Could you check a few things on this model? Use its own coordinates, in mm. Face numbers are marked on the shaded views. A direction names the side the tool comes from. Give positions to 0.01 mm unless a question says otherwise; leave off trailing zeros. Loops run counter-clockwise (first coordinate to the right, second up) from the corner with the lowest first, then second, coordinate; pieces in that order, holes last. Notation, with made-up numbers: (86.25, 18.25) - (139.25, 18.25) arc R11 cw to (139.25, 36.25) - close; hole circle Ø1 at (-38, 79.5). An arc over 180 degrees is marked (long way). Write each question's results on one line, items separated by ' | '. Start each with the question number.
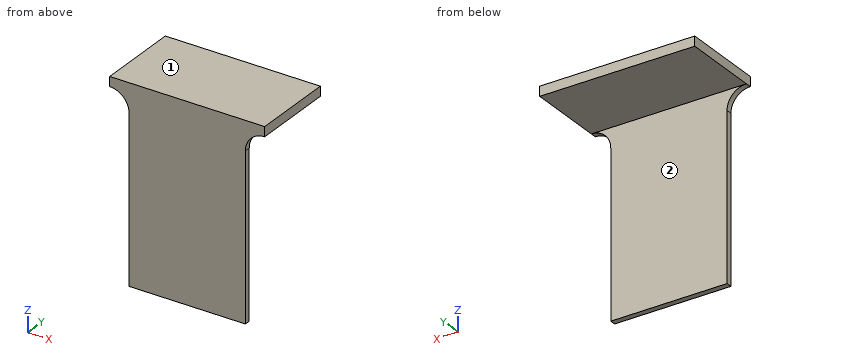
```python
from build123d import *

# Parameters (mm, degrees)
SKETCH_1_W           = 60
SKETCH_1_H           = 100
EXTRUDE_1_DEPTH      = 3
EXTRUDE_2_DEPTH      = 40
EXTRUDE_2_DEPTH_BACK = 3
SKETCH_2_W           = 80
SKETCH_2_H           = 5
FILLET_1_R           = 10


with BuildPart() as part:
    # Эскиз1 → Бобышка-Вытянуть1 (new body)
    with BuildSketch(Plane(origin=(0, 0, 0), x_dir=(1, 0, 0), z_dir=(0, 1, 0))):
        Rectangle(SKETCH_1_W, SKETCH_1_H)
    extrude(amount=EXTRUDE_1_DEPTH)

    # Эскиз2 → Бобышка-Вытянуть2 (add, two sides: drawn at the far end of the back side and taken through both)
    with BuildSketch(Plane(origin=(0, 3, 0), x_dir=(1, 0, 0), z_dir=(0, 1, 0)).offset(-EXTRUDE_2_DEPTH_BACK)):
        with Locations((0, -47.5)):
            Rectangle(SKETCH_2_W, SKETCH_2_H)
    extrude(amount=EXTRUDE_2_DEPTH + EXTRUDE_2_DEPTH_BACK)

    # Скругление1
    fillet_1_edges = [part.edges().sort_by_distance(p)[0] for p in [
        (30, 1.5, 45),
        (-30, 1.5, 45),
    ]]
    fillet(fillet_1_edges, radius=FILLET_1_R - 0.0001)  # a hair under: the kernel refuses the full size


solid = part.part
```
Q1. Which directions (+Z, -Z, +X, -X, +Y, -Y) give clear straight access to the entire face, cutting with the end or side of a thin tool? Please do the marked faces 1 and 2.
Q2. I want a section at C-C, the plane z = 26.5. List the corners of the cut face in (x, y) for me, then the cut area to 3 significant figures.
Q3. I need wall thicknesses on L1, parallel to Z at x = 29.5, y = 36.5; L2, parallel to Y at x = -7.5, z = 1. Which ranges of each line are inside material? Lowest first, please. Write a range as from..to.
Q4. I want a section at B-B, the plane y = 39.5. List the corners of the cut face in (x, z) for me.
Q5. I want a section at A-A, the plane x = 0. List the corners of the cut face in (y, z) for me.
Q6. I'm going to push flat-ended pins straight in: pin 1 Ø2 at (x, z) = (13, -28.5) entering from -Y; pin 2 Ø6 at (x, y) = (-17.5, 16) entering from -Z; pin 3 Ø3.5 at (y, z) = (2, 12) entering from +X; pin 4 Ø8 at (x, z) = (-7.5, -2) entering from +Y. Where does each tip first touch, or does it pass through?
Conclusion:
1) face 1: +Z, +X, -X, +Y, -Y | face 2: -Z, +X, -X, +Y
2) outline: (-30, 0) - (30, 0) - (30, 3) - (-30, 3) - close | area: 180 mm^2
3) L1: 45..50 | L2: 0..3
4) outline: (-40, 45) - (40, 45) - (40, 50) - (-40, 50) - close
5) outline: (0, -50) - (3, -50) - (3, 45) - (43, 45) - (43, 50) - (0, 50) - close
6) pin 1: y = 0 | pin 2: z = 45 | pin 3: x = 30 | pin 4: y = 3
